For this review, use the dimensioned drawing (mm, ordinates from the lowest corner) and the shaded views. A direction names the side the tool comes from. Round coordinates to 2 decimals unless told otherwise and drop trailing zeros. Loops run counter-clockwise (first coordinate to the right, second up) from the corner with the lowest first, then second, coordinate; pieces in that order, holes last. Notation, with made-up numbers: M 22,-34.5 L 61,-34.5 A23 ccw 61,-23.5 Z; hole C 5.25,42 d8. An arc over 180 degrees is marked long. One line per item, written item: value. Start each with the question number.
Item 1: Clearance check with flat-ended pins moving along their axes: pin 1 (3.5 mm diameter, centred on x = 25.5, y = 57.5, fed in from -Z); pin 2 (1.5 mm diameter, centred on y = 56.5, z = 10, fed in from +X); pin 3 (2.5 mm diameter, centred on x = 24.5, z = 44.5, fed in from -Y). State where each tip first meets the part, or that it passes through.
Item 2: We need section B-B (x = 26). Write out the cut boundary in (y, z).
Item 3: For the marked faces 5 and 6, list the 3-axis set-ups (+Z, -Z, +X, -X, +Y, -Y) from which the entire face can be reached by the end or side of a thin tool; tool diameter is ignored.
Item 4: We need section C-C (z = 79). Write out the cut boundary in (x, y), then the cut area to 3 significant figures.
Item 5: Mouldability with a two-part tool opening along Z and no side actions: class the marked faces 1, 2, 3 and 4 as released by +Z, released by -Z, zero draft, split by the parting line, or undercut.
Item 6: For line 1 along Y through (x, z) = (2.75, 45); line 2 along Y through (x, z) = (26, 45); line 3 along X through (y, z) = (70, 63), list the stretches that pass through material, from the lowest coordinate up.
Item 7: We need section D-D (y = 81). Write out the cut boundary in (x, z).
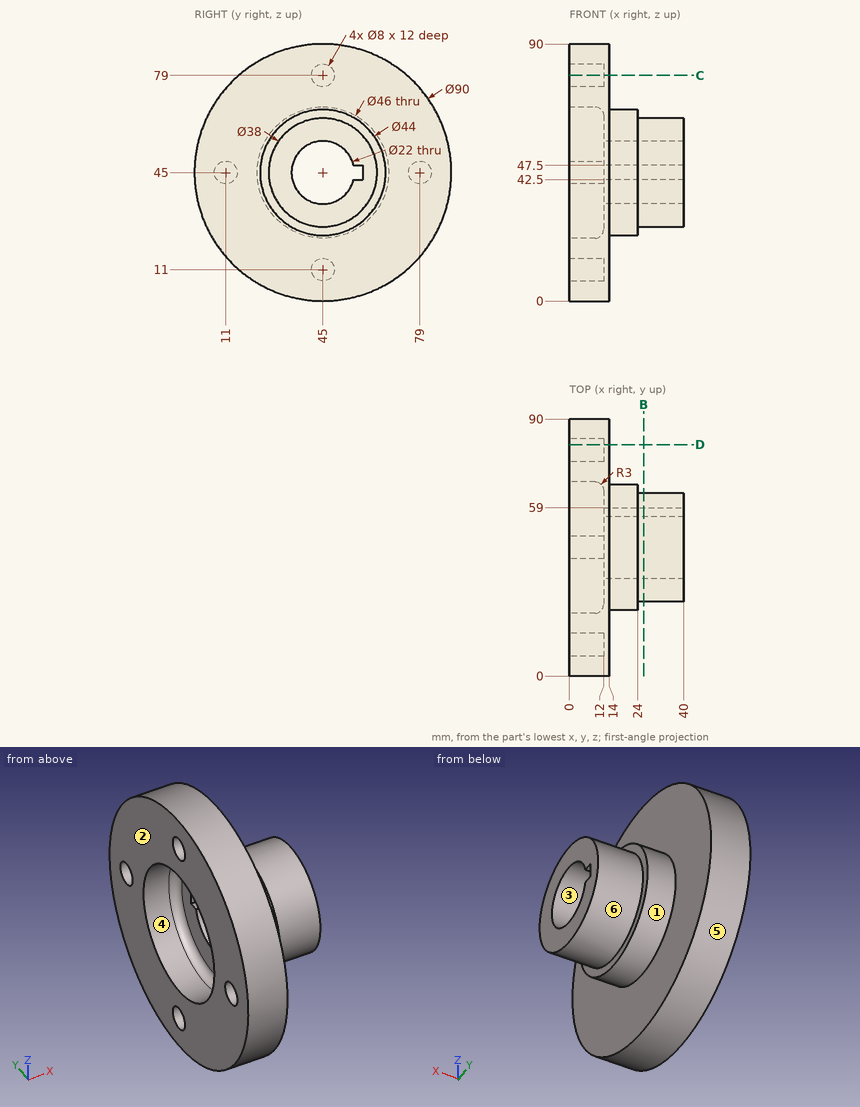
A:
1. pin 1: z = 26.31
1. pin 2: x = 14
1. pin 3: y = 23
2. outline: C 45,45 d38; hole M 55.71,42.5 L 59,42.5 L 59,47.5 L 55.71,47.5 A11 ccw long Z
3. face 5: +X, -X
3. face 6: +X
4. outline: M 0,15.52 L 14,15.52 L 14,74.48 L 0,74.48 L 0,49 L 12,49 L 12,41 L 0,41 Z
4. area: 729 mm2
5. face 1: split by the parting line
5. face 2: zero draft
5. face 3: undercut
5. face 4: undercut
6. line 1: 0 to 7, 15 to 22, 68 to 75, 83 to 90
6. line 2: 26 to 34, 59 to 64
6. line 3: 0 to 14
7. outline: M 0,18 L 14,18 L 14,72 L 0,72 L 0,48.46 L 12,48.46 L 12,41.54 L 0,41.54 Z
